Design review of the part built by this model. Coordinates are the model's own, in mm. Coordinates: 2 decimals unless noted, no trailing zeros. Loops run counter-clockwise (first coordinate to the right, second up) from the corner with the lowest first, then second, coordinate; pieces in that order, holes last.
from build123d import *

# Parameters (mm, degrees)
ESQUISSE1_R               = 1.7
T_LE_DE_BASE_PLI_E1_DEPTH = 0.5


# Sheet-metal steps are written as plain solids
with BuildPart() as part:
    # Esquisse1 → Tôle de base pliée1 (new body)
    with BuildSketch(Plane(origin=(0, 0, 0), x_dir=(1, 0, 0), z_dir=(0, 1, 0))):
        with BuildLine():
            Line((-35, -15), (35, -15))
            Line((35, -15), (35, -5.6))
            Line((35, -5.6), (-11.845934077, -5.6))
            ThreePointArc((-11.845934077, -5.6), (-20, 0), (-11.845934077, 5.6))
            Line((-11.845934077, 5.6), (35, 5.6))
            Line((35, 5.6), (35, 15))
            Line((35, 15), (-35, 15))
            Line((-35, 15), (-35, -15))
        make_face()
        with Locations(Location((30, 10, 0), (0, 0, 270))):
            Circle(ESQUISSE1_R, mode=Mode.SUBTRACT)
        with Locations(Location((30, -10, 0), (0, 0, 90))):
            Circle(ESQUISSE1_R, mode=Mode.SUBTRACT)
        with Locations(Location((-30, -10, 0), (0, 0, 270))):
            Circle(ESQUISSE1_R, mode=Mode.SUBTRACT)
        with Locations(Location((-30, 10, 0), (0, 0, 90))):
            Circle(ESQUISSE1_R, mode=Mode.SUBTRACT)
    extrude(amount=-T_LE_DE_BASE_PLI_E1_DEPTH)


solid = part.part
Q1. Take a section at A-A, the plane z = 10. Write out the cut boundary in (x, y).
Q2. Take a section at B-B, the plane x = 23. Write out the cut boundary in (y, z).
Q3. Take a section at C-C, the plane x = 30. Write out the cut boundary in (y, z).
Q4. The part is to be moulded in two halves that separate along X. For faces 1 (the cylindrical face through (28.34, -0.25, -10.37)), 2 (the flat face through (0, 0, 6)), 3 (the cylindrical face through (-31.66, -0.25, 9.63)), say which applies: pulls with the +X half, pulls with the -X half, needs draft (parallel to the pull), parting line crosses it, or undercut.
Q5. Take a section at D-D, the plane y = -0.25. Write out the cut boundary in (x, z), then the cut area to 3 significant figures.
Q6. For line 1 (X direction, y = -0.3, z = 10); line 2 (Z direction, x = 28, y = -0.3); line 3 (Z direction, x = -14, y = -0.3), list the stretches that pass through material, from the lowest coordinate up.
Q7. Clearance check with a flat-ended pin moving along its axis: pin 1 Ø12 at (x, z) = (5, -0.5) entering from -Y. State where the tip first meets the part, or that it passes through.
Entries:
1. outline: (-35, -0.5) - (-31.7, -0.5) - (-31.7, 0) - (-35, 0) - close; (-28.3, -0.5) - (28.3, -0.5) - (28.3, 0) - (-28.3, 0) - close; (31.7, -0.5) - (35, -0.5) - (35, 0) - (31.7, 0) - close
2. outline: (-0.5, -15) - (0, -15) - (0, -5.6) - (-0.5, -5.6) - close; (-0.5, 5.6) - (0, 5.6) - (0, 15) - (-0.5, 15) - close
3. outline: (-0.5, -15) - (0, -15) - (0, -11.7) - (-0.5, -11.7) - close; (-0.5, -8.3) - (0, -8.3) - (0, -5.6) - (-0.5, -5.6) - close; (-0.5, 5.6) - (0, 5.6) - (0, 8.3) - (-0.5, 8.3) - close; (-0.5, 11.7) - (0, 11.7) - (0, 15) - (-0.5, 15) - close
4. face 1: undercut
4. face 2: needs draft
4. face 3: undercut
5. outline: (-35, -15) - (35, -15) - (35, -5.6) - (-11.85, -5.6) arc R6 cw (long way) to (-11.85, 5.6) - (35, 5.6) - (35, 15) - (-35, 15) - close; hole circle Ø3.4 at (-30, -10); hole circle Ø3.4 at (-30, 10); hole circle Ø3.4 at (30, -10); hole circle Ø3.4 at (30, 10)
5. area: 1,460 mm2
6. line 1: x = -35 to -31.7, -28.3 to 28.3, 31.7 to 35
6. line 2: z = -15 to -5.6, 5.6 to 15
6. line 3: z = -15 to -6, 6 to 15
7. pin 1: stops at y = -0.5
